The listing builds one solid part. Answer for the finished solid, in the listing's coordinates (mm). Round coordinates to 2 decimals unless told otherwise and drop trailing zeros. Order: outer loops, then holes, each group sorted by start corner. A loop starts at its lowest first (then second) coordinate and runs counter-clockwise, first axis right, second up. Notation, with made-up numbers: (41.5, 34) - (94.5, 34) arc R7 ccw to (94.5, 46) - close; hole circle Ø9 at (81, 32.25). An arc over 180 degrees is marked (long way). One line per item, written item: value. Start each with the question number.
1. Section B-B, the plane z = 51.5 is taken. Give the vertices of the cut face in (x, y), then the cut area to 3 significant figures.
2. Section A-A, the plane y = -26.95 is taken. Count the separate pieces of the cut face and the enclosed holes in it, then the cut area to 3 significant figures.
3. Straight lines are drawn through the part: line 1 (X direction, y = -26.75, z = 171.5); line 2 (Z direction, x = -26.5, y = -25.5); line 3 (X direction, y = -26.65, z = 70.5). For each, find the intervals that lie inside material, in ascending order.
4. Flat-ended cylindrical pins translate along their axes: P1, Ø1.9, axis at x = 23.85, z = 170.25, coming from the -Y side; P2, Ø5, axis at x = 23.85, z = 112.25, coming from the -Y side; P3, Ø1, axis at y = -26.5, z = 36, coming from the +X side. Find the tip coordinate at first contact, or state that the pin passes through.
from build123d import *

# Parameters (mm, degrees)
BOSS_EXTRUDE1_DEPTH = 203.2
SKETCH3_R           = 1.5875
CUT_EXTRUDE1_DEPTH  = 209.029529299
SKETCH4_R           = 1.5875
CUT_EXTRUDE2_DEPTH  = 209.029529299


with BuildPart() as part:
    # Sketch2 → Boss-Extrude1 (new body)
    with BuildSketch(Plane.XY):
        with BuildLine():
            Line((-44.45, -24.593444248), (44.45, -24.593444248))
            ThreePointArc((44.45, -24.593444248), (43.515559877, -26.211372506), (42.522255607, -27.793844248))
            Line((42.522255607, -27.793844248), (-42.522255607, -27.793844248))
            ThreePointArc((-42.522255607, -27.793844248), (-43.515559877, -26.211372506), (-44.45, -24.593444248))
        make_face()
    extrude(amount=BOSS_EXTRUDE1_DEPTH)

    # Sketch3 → Cut-Extrude1 (cut, through all)
    with BuildSketch(Plane(origin=(0, -24.593444248, 0), x_dir=(1, 0, 0), z_dir=(0, 1, 0))):
        with Locations(Location((16.401757706, -19.478925293, 0), (0, 0, 270))):
            Circle(SKETCH3_R)
        with Locations(Location((-26.778242294, -70.278925293, 0), (0, 0, 270))):
            Circle(SKETCH3_R)
        with Locations(Location((21.137926992, -71.421925293, 0), (0, 0, 270))):
            Circle(SKETCH3_R)
        with Locations(Location((-11.538242294, -19.478925293, 0), (0, 0, 270))):
            Circle(SKETCH3_R)
    extrude(amount=-CUT_EXTRUDE1_DEPTH, mode=Mode.SUBTRACT)

    # Sketch4 → Cut-Extrude2 (cut, through all)
    with BuildSketch(Plane(origin=(0, -24.593444248, 0), x_dir=(1, 0, 0), z_dir=(0, 1, 0))):
        with Locations(Location((-25.152417206, -170.253365494, 0), (0, 0, 270))):
            Circle(SKETCH4_R)
        with Locations(Location((23.847582794, -170.253365494, 0), (0, 0, 270))):
            Circle(SKETCH4_R)
        with Locations(Location((23.847582794, -112.253365494, 0), (0, 0, 270))):
            Circle(SKETCH4_R)
        with Locations(Location((-25.152417206, -112.253365494, 0), (0, 0, 270))):
            Circle(SKETCH4_R)
    extrude(amount=-CUT_EXTRUDE2_DEPTH, mode=Mode.SUBTRACT)


solid = part.part
Answer list:
1. outline: (-44.45, -24.59) arc R50.8 ccw to (-42.52, -27.79) - (42.52, -27.79) arc R50.8 ccw to (44.45, -24.59) - close
1. area: 279 mm²
2. separate pieces: 1
2. enclosed holes: 8
2. area: 17,400 mm²
3. line 1: x = -43.19 to -26.14, -24.17 to 22.86, 24.83 to 43.19
3. line 2: z = 0 to 68.72, 71.84 to 111.41, 113.09 to 169.41, 171.09 to 203.2
3. line 3: x = -43.25 to -28.35, -25.21 to 19.85, 22.43 to 43.25
4. P1: passes through
4. P2: stops at y = -27.79
4. P3: stops at x = 43.64
